Input: part model. Units: mm. Frame: model coordinates. Coordinates: 2 decimals unless noted, no trailing zeros. Order: outer loops, then holes, each group sorted by start corner. A loop starts at its lowest first (then second) coordinate and runs counter-clockwise, first axis right, second up.
from build123d import *

# Parameters (mm, degrees)
F0_W     = 609.6
F0_H     = 609.6
F0_R     = 50.8
F0_R_2   = 3.175
F1_DEPTH = 25.4
F2_SIZE  = 2.8575


with BuildPart() as f1:
    # F0 (on Top) → F1 (new body)
    with BuildSketch(Plane.XY):
        with Locations((0, -30.747368)):
            Rectangle(F0_W, F0_H)
        with Locations((-228.6, -252.997368)):
            Circle(F0_R, mode=Mode.SUBTRACT)
        with Locations((-228.6, -75.197368)):
            Circle(F0_R, mode=Mode.SUBTRACT)
        with Locations((-76.2, -164.097368)):
            Circle(F0_R, mode=Mode.SUBTRACT)
        with Locations((76.2, -252.997368)):
            Circle(F0_R, mode=Mode.SUBTRACT)
        with Locations((76.2, -75.197368)):
            Circle(F0_R, mode=Mode.SUBTRACT)
        with Locations((228.6, -164.097368)):
            Circle(F0_R, mode=Mode.SUBTRACT)
        with Locations((-228.6, 102.602632)):
            Circle(F0_R, mode=Mode.SUBTRACT)
        with Locations((-76.2, 13.702632)):
            Circle(F0_R, mode=Mode.SUBTRACT)
        with Locations((-76.2, 191.502632)):
            Circle(F0_R, mode=Mode.SUBTRACT)
        with Locations((-101.6, 261.352632)):
            Circle(F0_R_2, mode=Mode.SUBTRACT)
        with Locations((76.2, 102.602632)):
            Circle(F0_R, mode=Mode.SUBTRACT)
        with Locations((228.6, 13.702632)):
            Circle(F0_R, mode=Mode.SUBTRACT)
        with Locations((101.6, 261.352632)):
            Circle(F0_R_2, mode=Mode.SUBTRACT)
        with Locations((228.6, 191.502632)):
            Circle(F0_R, mode=Mode.SUBTRACT)
    extrude(amount=F1_DEPTH)

    # F2
    f2_edges = [f1.edges().sort_by_distance(p)[0] for p in [
        (-25.4, -164.097368, 12.7),
        (-127, -164.097368, 0),
        (-127, -164.097368, 25.4),
        (-25.4, 13.702632, 12.7),
        (-127, 13.702632, 0),
        (-127, 13.702632, 25.4),
        (-177.8, 102.602632, 12.7),
        (-279.4, 102.602632, 0),
        (-279.4, 102.602632, 25.4),
        (-25.4, 191.502632, 12.7),
        (-127, 191.502632, 0),
        (-127, 191.502632, 25.4),
        (127, 102.602632, 12.7),
        (25.4, 102.602632, 0),
        (25.4, 102.602632, 25.4),
        (279.4, 191.502632, 12.7),
        (177.8, 191.502632, 0),
        (177.8, 191.502632, 25.4),
        (279.4, 13.702632, 12.7),
        (177.8, 13.702632, 0),
        (177.8, 13.702632, 25.4),
        (127, -75.197368, 12.7),
        (25.4, -75.197368, 0),
        (25.4, -75.197368, 25.4),
        (-177.8, -75.197368, 12.7),
        (-279.4, -75.197368, 0),
        (-279.4, -75.197368, 25.4),
        (-177.8, -252.997368, 12.7),
        (-279.4, -252.997368, 0),
        (-279.4, -252.997368, 25.4),
        (127, -252.997368, 12.7),
        (25.4, -252.997368, 0),
        (25.4, -252.997368, 25.4),
        (279.4, -164.097368, 12.7),
        (177.8, -164.097368, 0),
        (177.8, -164.097368, 25.4),
    ]]
    chamfer(f2_edges, length=F2_SIZE)


solid = f1.part
Item 1: Cut plane B-B on z = 11.75. Count the separate pieces of the cut face and the enclosed holes in it, then the cut area to 3 significant figures.
Response values:
separate pieces: 1
enclosed holes: 14
area: 274,000 mm2
Item 2: Cut plane A-A on x = -76.2. Return loops of the section in (y, z), then the cut area to 3 significant figures.
Response values:
outline: (-335.55, 0) - (-217.75, 0) - (-214.9, 2.86) - (-214.9, 22.54) - (-217.75, 25.4) - (-335.55, 25.4) - close; (-113.3, 2.86) - (-110.44, 0) - (-39.95, 0) - (-37.1, 2.86) - (-37.1, 22.54) - (-39.95, 25.4) - (-110.44, 25.4) - (-113.3, 22.54) - close; (64.5, 2.86) - (67.36, 0) - (137.85, 0) - (140.7, 2.86) - (140.7, 22.54) - (137.85, 25.4) - (67.36, 25.4) - (64.5, 22.54) - close; (242.3, 2.86) - (245.16, 0) - (274.05, 0) - (274.05, 25.4) - (245.16, 25.4) - (242.3, 22.54) - close
area: 7,690 mm2
Item 3: Pin query (flat end, axial travel): pin 1 Ø1 at (x, y) = (138, 166.5) entering from -Z. Return the tip coordinate at first contact, or that it passes through.
Response values:
pin 1: stops at z = 0
Item 4: Ray query, probe 1 along X at (y, z) = (-160, 10.5); probe 2 along Y at (x, z) = (-230, 22); probe 3 along X at (y, z) = (-75.5, 19). Return the intervals inside material, ascending.
Response values:
probe 1: x = -304.8 to -126.83, -25.57 to 177.97, 279.23 to 304.8
probe 2: y = -335.55 to -303.78, -202.22 to -125.98, -24.42 to 51.82, 153.38 to 274.05
probe 3: x = -304.8 to -279.4, -177.8 to 25.4, 127 to 304.8
Item 5: Draft query along Y for faces 1 (the face through (-4, -335.547, 13)), 2 (the face through (-304.8, -35, 13)), 3 (the face through (-180.146, -237.738, 12.562)). Return one class per face: pulls with the +Y half, pulls with the -Y half, needs draft (parallel to the pull), parting line crosses it, or undercut.
Response values:
face 1: pulls with the -Y half
face 2: needs draft
face 3: undercut
